For this review, take the finished solid that the model builds, in its own axes (mm). A direction names the side the tool comes from. Give positions to 0.01 mm unless a question says otherwise; leave off trailing zeros. Order: outer loops, then holes, each group sorted by start corner. A loop starts at its lowest first (then second) coordinate and runs counter-clockwise, first axis right, second up.
Item 1: For probe 1 along X at (y, z) = (-0.85, 0); probe 2 along Z at (x, y) = (-41.5, -0.85); probe 3 along X at (y, z) = (-1.15, 0.45), list the stretches that pass through material, from the lowest coordinate up.
Item 2: For P1, Ø2, axis at x = -53, z = 2, coming from the +Y side, flat-tipped, find the tip position at first contact; note if it passes through.
Item 3: Machinability: for faces 1 (the flat face through (-51.646, 1.173, 1.16)), 2 (the flat face through (-48, 0, 1.65)), 3 (the flat face through (-48, 0, -1.65)), which of the approach directions +Z, -Z, +X, -X, +Y, -Y give a long, thin tool a straight path to every point of the face, cutting with its end or side? Answer none if there is none.
Item 4: The part is to be moulded in two halves that separate along Z. For faces 4 (the flat face through (-45, 1.65, 0)), 5 (the flat face through (-51.646, -1.16, 1.173)), 6 (the flat face through (-51.646, -1.173, -1.16)), 7 (the cylindrical face through (-42.984, -0.023, -0.303)), say which applies: released by +Z, released by -Z, zero draft, split by the parting line, or undercut.
Item 5: Consider section C-C (x = -48). Give the boundary of the cut face in (y, z).
Item 6: Consider section D-D (y = -0.5). Give the boundary of the cut face in (x, z).
Item 7: Consider section B-B (y = 0.15). Give the boundary of the cut face in (x, z), plus the area to 3 significant figures.
Item 8: Consider section A-A (z = 0). Give the boundary of the cut face in (x, y), plus the area to 3 significant figures.
```python
from build123d import *

# Parameters (mm, degrees)
SKETCH1_R                = 30
SKETCH1_R_2              = 14
BOSS_EXTRUDE1_DEPTH      = 18
BOSS_EXTRUDE2_DEPTH      = 45
SKETCH3_R                = 15
BOSS_EXTRUDE3_DEPTH      = 22
BOSS_EXTRUDE4_REACH      = 112.675
SKETCH4_W                = 33
SKETCH4_H                = 33
FILLET1_R                = 5
FILLET7_R                = 1.5
SCALA2_SCALE             = 0.1
SCHIZZO1_W               = 13.938376935
SCHIZZO1_H               = 12.715061938
TAGLIO_ESTRUSIONE1_DEPTH = 0.15
SCHIZZO2_W               = 8.711485585
SCHIZZO2_H               = 10.583528232
TAGLIO_ESTRUSIONE2_DEPTH = 0.15


with BuildPart() as part:
    # Sketch1 → Boss-Extrude1 (new, symmetric)
    with BuildSketch(Plane(origin=(0, 0, 0), x_dir=(1, 0, 0), z_dir=(0, 1, 0))):
        with Locations(Location((0, 0, 0), (0, 0, 270))):
            Circle(SKETCH1_R)
        with Locations(Location((0, 0, 0), (0, 0, 270))):
            Circle(SKETCH1_R_2, mode=Mode.SUBTRACT)
    extrude(amount=BOSS_EXTRUDE1_DEPTH, both=True)

    # Sketch4 → Boss-Extrude4 (add, up to next)
    with BuildSketch(Plane(origin=(-75, 0, 0), x_dir=(0, 0, -1), z_dir=(1, 0, 0)), mode=Mode.PRIVATE) as boss_extrude4_sk1:
        Rectangle(SKETCH4_W, SKETCH4_H)
    boss_extrude4_tool1 = extrude(boss_extrude4_sk1.sketch, amount=BOSS_EXTRUDE4_REACH, mode=Mode.PRIVATE) - part.part


with BuildPart() as body_2:
    # Sketch2 → Boss-Extrude2 (new body)
    with BuildSketch(Plane(origin=(-120, 0, 0), x_dir=(0, 0, -1), z_dir=(1, 0, 0))):
        Polygon((-16.5, 6.834523779), (-16.5, -6.834523779), (-6.834523779, -16.5), (6.834523779, -16.5), (16.5, -6.834523779), (16.5, 6.834523779), (6.834523779, 16.5), (-6.834523779, 16.5), align=None)
    extrude(amount=BOSS_EXTRUDE2_DEPTH)

    # Sketch3 → Boss-Extrude3 (add)
    with BuildSketch(Plane(origin=(-120, 0, 0), x_dir=(0, 0, -1), z_dir=(1, 0, 0))):
        Circle(SKETCH3_R)
    extrude(amount=-BOSS_EXTRUDE3_DEPTH)


with BuildPart() as part_1:
    add(part.part)

    add(body_2.part)  # Boss-Extrude4 merges body 2
    add(boss_extrude4_tool1.solids().sort_by_distance((-75, 0, 0))[0])

    # Fillet1
    fillet1_edges = [part_1.edges().sort_by_distance(p)[0] for p in [
        (-75, 11.66726189, 11.66726189),
        (-75, -11.66726189, 11.66726189),
        (-75, -11.66726189, -11.66726189),
        (-75, 11.66726189, -11.66726189),
    ]]
    fillet(fillet1_edges, radius=FILLET1_R)

    # Fillet7
    fillet7_edges = [part_1.edges().sort_by_distance(p)[0] for p in [
        (-30, -16.5, 0),
        (-30, 16.5, 0),
    ]]
    fillet(fillet7_edges, radius=FILLET7_R - 0.0001)  # a hair under: the kernel refuses the full size


with BuildPart() as part_2:
    # Scala2: scaled about (-46.241792436, -2e-09, 0)
    add(part_1.part.scale(SCALA2_SCALE).moved(Location((-41.617613192, -2e-09, 0))))

    # Schizzo1 → Taglio-Estrusione1 (cut)
    with BuildSketch(Plane(origin=(0, 1.8, 0), x_dir=(1, 0, 0), z_dir=(0, 1, 0))):
        with Locations((-40.78597266, -0.750670566)):
            Rectangle(SCHIZZO1_W, SCHIZZO1_H)
    extrude(amount=-TAGLIO_ESTRUSIONE1_DEPTH, mode=Mode.SUBTRACT)

    # Schizzo2 → Taglio-Estrusione2 (cut)
    with BuildSketch(Plane.XZ.offset(1.8)):
        with Locations((-41.379095083, -0.12974553)):
            Rectangle(SCHIZZO2_W, SCHIZZO2_H)
    extrude(amount=-TAGLIO_ESTRUSIONE2_DEPTH, mode=Mode.SUBTRACT)


solid = part_2.part
```
Resolved:
1. probe 1: x = -55.82 to -43.02, -40.22 to -38.62
1. probe 2: z = -3 to -1.4, 1.4 to 3
1. probe 3: x = -55.82 to -42.94, -40.29 to -38.65
2. P1: stops at y = 1.33
3. face 1: +Z, -X, +Y
3. face 2: +Z, -X, +Y, -Y
3. face 3: -Z, -X, +Y, -Y
4. face 4: zero draft
4. face 5: released by +Z
4. face 6: released by -Z
4. face 7: undercut
5. outline: (-1.65, -1.65) - (1.65, -1.65) - (1.65, 1.65) - (-1.65, 1.65) - close
6. outline: (-55.82, -1.41) - (-53.62, -1.41) - (-53.62, -1.65) - (-44.12, -1.65) arc R3 ccw (long way) to (-44.12, 1.65) - (-53.62, 1.65) - (-53.62, 1.41) - (-55.82, 1.41) - close; hole circle Ø2.8 at (-41.62, 0)
7. outline: (-55.82, -1.49) - (-53.62, -1.49) - (-53.62, -1.65) - (-44.12, -1.65) arc R3 ccw (long way) to (-44.12, 1.65) - (-53.62, 1.65) - (-53.62, 1.49) - (-55.82, 1.49) - close; hole circle Ø2.8 at (-41.62, 0)
7. area: 58.9 mm2
8. outline: (-55.82, -1.5) - (-53.62, -1.5) - (-53.62, -1.65) - (-43.02, -1.65) - (-43.02, 1.65) - (-53.62, 1.65) - (-53.62, 1.5) - (-55.82, 1.5) - close; (-40.22, -1.65) - (-38.62, -1.65) - (-38.62, 1.65) - (-40.22, 1.65) - close
8. area: 46.9 mm2
